Check sheet for the modelled part. Datum: model origin and axes. Units: mm. A direction names the side the tool comes from. Coordinates: 2 decimals unless noted, no trailing zeros. Write each question's results on one line, items separated by ' | '. Start each with the question number.
from build123d import *

# Parameters (mm, degrees)
SKETCH_W      = 200
SKETCH_H      = 500
PAD_DEPTH     = 50
SKETCH001_R   = 52.5
SKETCH001_R_2 = 16
POCKET_DEPTH  = 1
FILLET_R      = 10


with BuildPart() as part:
    # Sketch (on XY_Plane of Origin) → Pad (new body)
    with BuildSketch(Plane.XY):
        Rectangle(SKETCH_W, SKETCH_H)
    extrude(amount=PAD_DEPTH)

    # Sketch001 (on Face6 of Pad) → Pocket (cut)
    with BuildSketch(Plane.XY.offset(50)):
        with Locations((0, 120)):
            Circle(SKETCH001_R)
        with Locations((0, -120)):
            Circle(SKETCH001_R)
        with Locations((-50, 0)):
            Circle(SKETCH001_R_2)
    extrude(amount=-POCKET_DEPTH, mode=Mode.SUBTRACT)

    # Fillet
    fillet_edges = [part.edges().sort_by_distance(p)[0] for p in [
        (-100, 0, 50),
    ]]
    fillet(fillet_edges, radius=FILLET_R)


solid = part.part
1) Thickness scan on probe 1 along Y at (x, z) = (0, 49.7); probe 2 along Z at (x, y) = (26, -101); probe 3 along X at (y, z) = (-99, 41.5). Record the ranges inside material, lowest first.
2) Gauge pin test, flat end, axial feed: P1, Ø9.5, axis at x = -45, y = 2, coming from the +Z side. Record the tip position at first contact, or that the pin passes through.
3) Release check for a two-part mould opening along Y. For faces 1 (the flat face through (-1, 121, 49)), 2 (the flat face through (100, -3, 25)), 3 (the flat face through (-1, -250, 25)) record: +Y half, -Y half, draft (parallel to the pull), parting line (faces both ways), or undercut.
4) Set-up check for faces 4 (the cylindrical face through (50.076, -104.23, 49.507)), 5 (the flat face through (-1, 4, 0)): record each of +Z, -Z, +X, -X, +Y, -Y from which the full face is reachable in a straight line by a thin tool's end or side.
Return value:
1) probe 1: y = -250 to -172.5, -67.5 to 67.5, 172.5 to 250 | probe 2: z = 0 to 49 | probe 3: x = -99.89 to 100
2) P1: stops at z = 49
3) face 1: undercut | face 2: draft | face 3: -Y half
4) face 4: +Z | face 5: -Z, +X, -X, +Y, -Y
